Model file for the job. Use its own axes, mm. A direction names the side the tool comes from. Coordinates: 2 decimals unless noted, no trailing zeros. Order: outer loops, then holes, each group sorted by start corner. A loop starts at its lowest first (then second) coordinate and runs counter-clockwise, first axis right, second up. Notation, with made-up numbers: M 76.25,29.5 L 125.25,29.5 A18 ccw 125.25,54.5 Z; hole C 22,3 d1. An arc over 180 degrees is marked long. Return JSON: item names as keys, results as strings.
```python
from build123d import *

# Parameters (mm, degrees)
F0_R      = 31.75
F0_R_2    = 29.21
F1_DEPTH  = 76.2
F2_R      = 31.75
F2_R_2    = 29.21
F3_DEPTH  = 76.2
F4_DEPTH  = 52.832
F5_DEPTH  = 44.45
F7_W      = 97.233793
F7_H      = 111.76
F8_DEPTH  = 2.032
F9_R      = 2.54
F10_DEPTH = 25.4


with BuildPart() as f1:
    # F0 (on Front) → F1 (new body, symmetric)
    with BuildSketch(Plane.XZ):
        Circle(F0_R)
        Circle(F0_R_2, mode=Mode.SUBTRACT)
    extrude(amount=F1_DEPTH, both=True)

    # F2 (on Right) → F3 (join)
    with BuildSketch(Plane.YZ):
        Circle(F2_R)
        Circle(F2_R_2, mode=Mode.SUBTRACT)
    extrude(amount=F3_DEPTH)

    # F0 (on Front) → F4 (cut, symmetric)
    with BuildSketch(Plane.XZ):
        Circle(F0_R_2)
    extrude(amount=F4_DEPTH, both=True, mode=Mode.SUBTRACT)

    # F2 (on Right) → F5 (cut)
    with BuildSketch(Plane.YZ):
        Circle(F2_R_2)
    extrude(amount=F5_DEPTH, mode=Mode.SUBTRACT)

    # F7 (on offset) → F8 (join, symmetric)
    with BuildSketch(Plane.XY.offset(-31.75)):
        with Locations((7.263103, 0)):
            Rectangle(F7_W, F7_H)
    extrude(amount=F8_DEPTH, both=True)

    # F9 (on face) → F10 (cut)
    with BuildSketch(Plane.XY.offset(-29.718)):
        with Locations((-36.273793, 50.8)):
            Circle(F9_R)
        with Locations((50.8, 50.8)):
            Circle(F9_R)
        with Locations((50.8, -50.8)):
            Circle(F9_R)
        with Locations((-36.273793, -50.8)):
            Circle(F9_R)
    extrude(amount=-F10_DEPTH, mode=Mode.SUBTRACT)


solid = f1.part
```
Item 1: Saw through at D-D (y = 0). Write the cut outline in (x, z), and give its area (3 significant figures).
Check result:
{"outline": "M -41.35,-33.78 L 55.88,-33.78 L 55.88,-31.75 L 76.2,-31.75 L 76.2,-29.21 L 0,-29.21 A29.21 cw 0,29.21 L 76.2,29.21 L 76.2,31.75 L 0,31.75 A31.75 ccw -11.18,-29.72 L -41.35,-29.72 Z", "area": "897 mm2"}
Item 2: Wall check: line 1 (Z direction, x = 48, y = 0); line 2 (Y direction, x = 50.8, z = -30.9); line 3 (Z direction, x = 32.5, y = -19.5). Give the ranges that are in metal, low to high.
Check result:
{"line 1": "z = -33.78 to -29.21, 29.21 to 31.75", "line 2": "y = -55.88 to -53.34, -48.26 to 48.26, 53.34 to 55.88", "line 3": "z = -33.78 to -29.72, -25.06 to -21.75, 21.75 to 25.06"}
Item 3: Saw through at A-A (y = 50.8). Write the cut outline in (x, z), and give its area (3 significant figures).
Check result:
{"outline": "M -41.35,-33.78 L -38.81,-33.78 L -38.81,-29.72 L -41.35,-29.72 Z; M -33.73,-33.78 L 48.26,-33.78 L 48.26,-29.72 L 11.18,-29.72 A31.75 ccw long -11.18,-29.72 L -33.73,-29.72 Z; M 53.34,-33.78 L 55.88,-33.78 L 55.88,-29.72 L 53.34,-29.72 Z; hole C 0,0 d58.42", "area": "810 mm2"}
Item 4: 3-axis set-ups, long thin cutter, end or side, ignore diameter. For faces 1 (the flat face through (7, 55.88, -32)), 2 (the cylindrical face through (46.033, 27.861, 8.774)), 3 (the flat face through (33, -33, -29.718)), 4 (the cylindrical face through (-23.4, -1.07, 21.46)), 5 (the flat face through (55.88, -1, -32)): which of +Z, -Z, +X, -X, +Y, -Y reach the whole face in a straight line?
Check result:
{"face 1": "-Z, +Y", "face 2": "+X", "face 3": "+X, -Y", "face 4": "none", "face 5": "-Z, +X"}
Item 5: Saw through at B-B (z = 0). Write the cut outline in (x, y), and give its area (3 significant figures).
Check result:
{"outline": "M -31.75,-76.2 L -29.21,-76.2 L -29.21,76.2 L -31.75,76.2 Z; M 29.21,-76.2 L 31.75,-76.2 L 31.75,-31.75 L 76.2,-31.75 L 76.2,-29.21 L 29.21,-29.21 Z; M 29.21,29.21 L 76.2,29.21 L 76.2,31.75 L 31.75,31.75 L 31.75,76.2 L 29.21,76.2 Z", "area": "852 mm2"}
Item 6: Saw through at C-C (x = 50.8). Write the cut outline in (y, z), and give its area (3 significant figures).
Check result:
{"outline": "M -55.88,-33.78 L -53.34,-33.78 L -53.34,-29.72 L -55.88,-29.72 Z; M -48.26,-33.78 L 48.26,-33.78 L 48.26,-29.72 L 11.18,-29.72 A31.75 ccw long -11.18,-29.72 L -48.26,-29.72 Z; M 53.34,-33.78 L 55.88,-33.78 L 55.88,-29.72 L 53.34,-29.72 Z; hole C 0,0 d58.42", "area": "869 mm2"}
Item 7: Pull direction Y, two halves, no side cores. Call faces 6 (the cylindrical face through (-34.908, -48.658, -31.722)), 7 (the flat face through (7, -55.88, -32)), 8 (the cylindrical face through (-33.927, 49.827, -31.722)), 9 (the flat face through (7, 1, -33.782)): +Y half, -Y half, draft (parallel to the pull), parting line (faces both ways), or undercut.
Check result:
{"face 6": "undercut", "face 7": "-Y half", "face 8": "undercut", "face 9": "draft"}
Item 8: Drop flat-ended pins along their axis: pin 1 Ø2 at (y, z) = (-5, -23.5) entering from -X; pin 2 Ø10 at (y, z) = (29, 5.5) entering from -X; pin 3 Ø2 at (x, z) = (18.5, -32.5) entering from -Y. Give the stop position or say it passes through.
Check result:
{"pin 1": "stops at x = -22.4", "pin 2": "stops at x = -31.75", "pin 3": "stops at y = -55.88"}
